Build history of the part. All positions in model axes, mm. Face numbers are marked on the shaded views. A direction names the side the tool comes from. Give positions to 0.01 mm unless a question says otherwise; leave off trailing zeros. Order: outer loops, then holes, each group sorted by start corner. A loop starts at its lowest first (then second) coordinate and runs counter-clockwise, first axis right, second up. Notation, with made-up numbers: M -34,-18 L -3,-18 A19 ccw -3,-13 Z; hole C 73.5,24 d11. An arc over 180 degrees is marked long. One line per item, written item: value.
from build123d import *
from OCP.BRepFilletAPI import BRepFilletAPI_MakeChamfer

# Parameters (mm, degrees)
BOSS_EXTRUDE1_DEPTH = 6.35
SKETCH2_R           = 1.15
CUT_EXTRUDE1_DEPTH  = 6.35
SKETCH3_W           = 0.5
SKETCH3_H           = 2.8
BOSS_EXTRUDE2_DEPTH = 7.25
SKETCH4_R           = 0.625
CUT_EXTRUDE2_DEPTH  = 16.25
CHAMFER1_SIZE       = 0.5
CHAMFER2_SIZE       = 0.5
CHAMFER2_SIZE2      = 0.08816349
SKETCH5_W           = 6.5
SKETCH5_H           = 2.5
SKETCH5_R           = 0.85
CUT_EXTRUDE4_DEPTH  = 0.5
FILLET1_R           = 1.5


with BuildPart() as part:
    # Sketch1 → Boss-Extrude1 (new body)
    with BuildSketch(Plane(origin=(0, 0, 0), x_dir=(1, 0, 0), z_dir=(0, 1, 0))):
        Polygon((9.35, 9.35), (9.75, 9), (16.75, 9), (20, 8.65), (20, 0), (0, 0), (0, 9.35), align=None)
    extrude(amount=BOSS_EXTRUDE1_DEPTH)

    # Sketch2 → Cut-Extrude1 (cut)
    with BuildSketch(Plane(origin=(0, 6.35, 0), x_dir=(1, 0, 0), z_dir=(0, 1, 0))):
        with Locations(Location((14.75, 2.45, 0), (0, 0, 270))):
            Circle(SKETCH2_R)
        with Locations(Location((5, 2.45, 0), (0, 0, 270))):
            Circle(SKETCH2_R)
    extrude(amount=-CUT_EXTRUDE1_DEPTH, mode=Mode.SUBTRACT)

    # Sketch3 → Boss-Extrude2 (add)
    with BuildSketch(Plane.XY):
        with Locations((2.25, 3.05)):
            Rectangle(SKETCH3_W, SKETCH3_H)
        with Locations((9.75, 3.05)):
            Rectangle(SKETCH3_W, SKETCH3_H)
        with Locations((17.25, 3.05)):
            Rectangle(SKETCH3_W, SKETCH3_H)
    extrude(amount=BOSS_EXTRUDE2_DEPTH)

    # Sketch4 → Cut-Extrude2 (cut)
    with BuildSketch(Plane.ZY.offset(-2)):
        with Locations((5.25, 3.05)):
            Circle(SKETCH4_R)
    extrude(amount=-CUT_EXTRUDE2_DEPTH, mode=Mode.SUBTRACT)

    # Chamfer1
    chamfer1_edges = [part.edges().sort_by_distance(p)[0] for p in [
        (2.25, 4.45, 7.25),
        (2.25, 1.65, 7.25),
        (9.75, 1.65, 7.25),
        (9.75, 4.45, 7.25),
        (17.25, 1.65, 7.25),
        (17.25, 4.45, 7.25),
    ]]
    chamfer(chamfer1_edges, length=CHAMFER1_SIZE)

    # Chamfer2: one chamfer whose edges measure the first distance from different faces: ONE call of the kernel's chamfer builder (chamfer() names one face for all edges)
    chamfer2_edges_1 = [part.edges().sort_by_distance(p)[0] for p in [
        (2.5, 3.05, 7.25),
    ]]
    chamfer2_side_1 = [part.faces().sort_by_distance(p)[0] for p in [
        (2.5, 3.05, 3.473122701),
    ]]
    chamfer2_edges_2 = [part.edges().sort_by_distance(p)[0] for p in [
        (2, 3.05, 7.25),
    ]]
    chamfer2_side_2 = [part.faces().sort_by_distance(p)[0] for p in [
        (2, 3.05, 3.473122701),
    ]]
    chamfer2_edges_3 = [part.edges().sort_by_distance(p)[0] for p in [
        (9.5, 3.05, 7.25),
    ]]
    chamfer2_side_3 = [part.faces().sort_by_distance(p)[0] for p in [
        (9.5, 3.05, 3.473122701),
    ]]
    chamfer2_edges_4 = [part.edges().sort_by_distance(p)[0] for p in [
        (10, 3.05, 7.25),
    ]]
    chamfer2_side_4 = [part.faces().sort_by_distance(p)[0] for p in [
        (10, 3.05, 3.473122701),
    ]]
    chamfer2_edges_5 = [part.edges().sort_by_distance(p)[0] for p in [
        (17, 3.05, 7.25),
    ]]
    chamfer2_side_5 = [part.faces().sort_by_distance(p)[0] for p in [
        (17, 3.05, 3.473122701),
    ]]
    chamfer2_edges_6 = [part.edges().sort_by_distance(p)[0] for p in [
        (17.5, 3.05, 7.25),
    ]]
    chamfer2_side_6 = [part.faces().sort_by_distance(p)[0] for p in [
        (17.5, 3.05, 3.473122701),
    ]]
    chamfer2 = BRepFilletAPI_MakeChamfer(part.part.solid().wrapped)
    for e in chamfer2_edges_1:
        chamfer2.Add(CHAMFER2_SIZE, CHAMFER2_SIZE2, e.wrapped, chamfer2_side_1[0].wrapped)  # the first distance lies on this face
    for e in chamfer2_edges_2:
        chamfer2.Add(CHAMFER2_SIZE, CHAMFER2_SIZE2, e.wrapped, chamfer2_side_2[0].wrapped)  # the first distance lies on this face
    for e in chamfer2_edges_3:
        chamfer2.Add(CHAMFER2_SIZE, CHAMFER2_SIZE2, e.wrapped, chamfer2_side_3[0].wrapped)  # the first distance lies on this face
    for e in chamfer2_edges_4:
        chamfer2.Add(CHAMFER2_SIZE, CHAMFER2_SIZE2, e.wrapped, chamfer2_side_4[0].wrapped)  # the first distance lies on this face
    for e in chamfer2_edges_5:
        chamfer2.Add(CHAMFER2_SIZE, CHAMFER2_SIZE2, e.wrapped, chamfer2_side_5[0].wrapped)  # the first distance lies on this face
    for e in chamfer2_edges_6:
        chamfer2.Add(CHAMFER2_SIZE, CHAMFER2_SIZE2, e.wrapped, chamfer2_side_6[0].wrapped)  # the first distance lies on this face
    add(Compound.cast(chamfer2.Shape()), mode=Mode.REPLACE)

    # Sketch5 → Cut-Extrude4 (cut)
    with BuildSketch(Plane(origin=(0, 6.35, 0), x_dir=(1, 0, 0), z_dir=(0, 1, 0))):
        with Locations((3.75, 8.1)):
            Rectangle(SKETCH5_W, SKETCH5_H)
        with Locations(Location((2.5, 8.49, 0), (0, 0, 270))):
            Circle(SKETCH5_R, mode=Mode.SUBTRACT)
        with Locations(Location((5.5, 8.49, 0), (0, 0, 270))):
            Circle(SKETCH5_R, mode=Mode.SUBTRACT)
    cut_extrude4 = extrude(amount=-CUT_EXTRUDE4_DEPTH, mode=Mode.SUBTRACT)

    # Mirror1: Cut-Extrude4 across plane
    add(cut_extrude4.mirror(Plane(origin=(0, 3.175, 0), x_dir=(0, 0, 1), z_dir=(0, -1, 0))), mode=Mode.SUBTRACT)

    # Fillet1
    fillet1_edges = [part.edges().sort_by_distance(p)[0] for p in [
        (0.5, 6.1, -6.85),
        (7, 6.1, -6.85),
        (0.5, 0.25, -6.85),
        (7, 0.25, -6.85),
    ]]
    fillet(fillet1_edges, radius=FILLET1_R)


solid = part.part
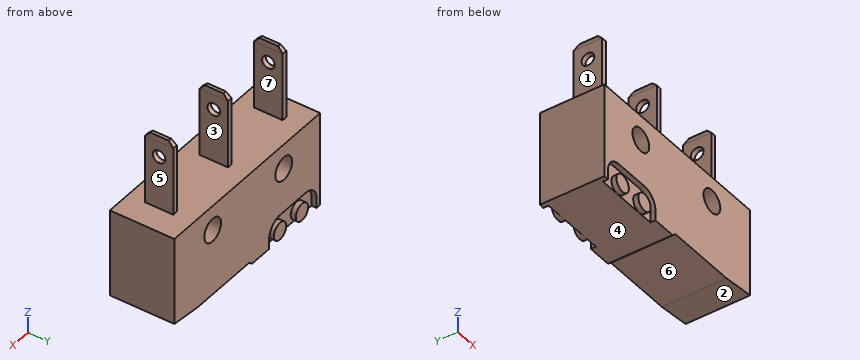
1) Tool access for the marked faces 4, 5, 6 and 7: list every direction of +Z, -Z, +X, -X, +Y, -Y with a clear straight run to the whole face (end or side of a thin tool).
Check values:
face 4: -Z, +X, -X, +Y, -Y
face 5: +Z, +X, +Y, -Y
face 6: -Z, +X, +Y, -Y
face 7: +Z, +Y, -Y
2) Drill centre lines: probe 1 along X at (y, z) = (3.5, 1.5); probe 2 along X at (y, z) = (1.5, -2.45); probe 3 along Z at (x, y) = (4, 6). Where is each one in solid material? Low to high. Write a range as from..to.
Check values:
probe 1: 2..2.5, 9.5..10, 17..17.5
probe 2: 0..3.85, 6.15..13.6, 15.9..20
probe 3: -6.85..-3.02, -1.88..0
3) Saw through at D-D, the plane z = 2.75. Write the cut outline in (x, y), then the cut area to 3 significant figures.
Check values:
outline: M 2,1.65 L 2.5,1.65 L 2.5,4.45 L 2,4.45 Z; M 9.5,1.65 L 10,1.65 L 10,4.45 L 9.5,4.45 Z; M 17,1.65 L 17.5,1.65 L 17.5,4.45 L 17,4.45 Z
area: 4.20 mm^2
4) Mould opens along X. For the marked faces 1, 2 and 3 say: released by +X, released by -X, zero draft, split by the parting line, or undercut.
Check values:
face 1: released by -X
face 2: released by +X
face 3: undercut
5) Pin check, flat tips, straight feed: pin 1 (3 mm diameter, centred on x = 2, z = 2.5, fed in from -Y); pin 2 (2 mm diameter, centred on y = 3, z = 3, fed in from +X); pin 3 (2 mm diameter, centred on y = 3, z = 3, fed in from -X). Stop position of each tip, or through.
Check values:
pin 1: y = 1.65
pin 2: x = 17.5
pin 3: x = 2
6) Saw through at A-A, the plane z = -2.45. Write the cut outline in (x, y), then the cut area to 3 significant figures.
Check values:
outline: M 0,0 L 3.85,0 L 3.85,6.35 L 0,6.35 Z; M 6.15,0 L 13.6,0 L 13.6,6.35 L 6.15,6.35 Z; M 15.9,0 L 20,0 L 20,6.35 L 15.9,6.35 Z
area: 97.8 mm^2
7) Saw through at B-B, the plane y = 1.25. Write the cut outline in (x, z).
Check values:
outline: M 0,-9.35 L 9.35,-9.35 L 9.75,-9 L 16.75,-9 L 20,-8.65 L 20,0 L 0,0 Z; hole C 5,-2.45 d2.3; hole C 14.75,-2.45 d2.3
8) Saw through at C-C, the plane x = 14.75. Write the cut outline in (y, z).
Check values:
outline: M 0,-9 L 6.35,-9 L 6.35,-3.6 L 0,-3.6 Z; M 0,-1.3 L 6.35,-1.3 L 6.35,0 L 0,0 Z
